Drawing for the job (mm, zero at the part's lowest x, y, z). A direction names the side the tool comes from. Give positions to 0.01 mm unless a question says otherwise; leave off trailing zeros. Order: outer loops, then holes, each group sorted by start corner. A loop starts at its lowest first (then second) coordinate and runs counter-clockwise, first axis right, second up. Notation, with made-up numbers: (43.25, 17.25) - (53.25, 17.25) arc R20 ccw to (53.25, 25.25) - close; hole circle Ø8 at (62.5, 49.25). An arc over 180 degrees is marked (long way). Use a Markdown table: item, result. Add a question column.
(1) Slice it at A-A (y = 12). Write the cut outline in (x, z) (1 decimal).
(2) Which spindle directions (+Z, -Z, +X, -X, +Y, -Y) get a long thin tool onto all of the face, cutting with end or side? Do the marked faces 1, 2 and 3. Say none if no direction does.
(3) Slice it at B-B (x = 4.45). Write the cut outline in (y, z) (1 decimal), then the cut area to 3 significant figures.
(4) Wall check: line 1 (Z direction, x = 0.5, y = 5.75) (1 decimal). Give the ranges that are in metal, low to high.
(5) Slice it at C-C (z = 4.45). Write the cut outline in (x, y) (1 decimal), then the cut area to 3 significant figures.
(6) Flat gauge pins, fed straight in: pin 1 (0.8 mm diameter, centred on y = 11, z = 4, fed in from +X) (1 decimal); pin 2 (0.8 mm diameter, centred on x = 1, y = 7, fed in from -Z); pin 3 (0.8 mm diameter, centred on x = 1, y = 7, fed in from +Z) (1 decimal). Where does each tip first touch, or does it go through?
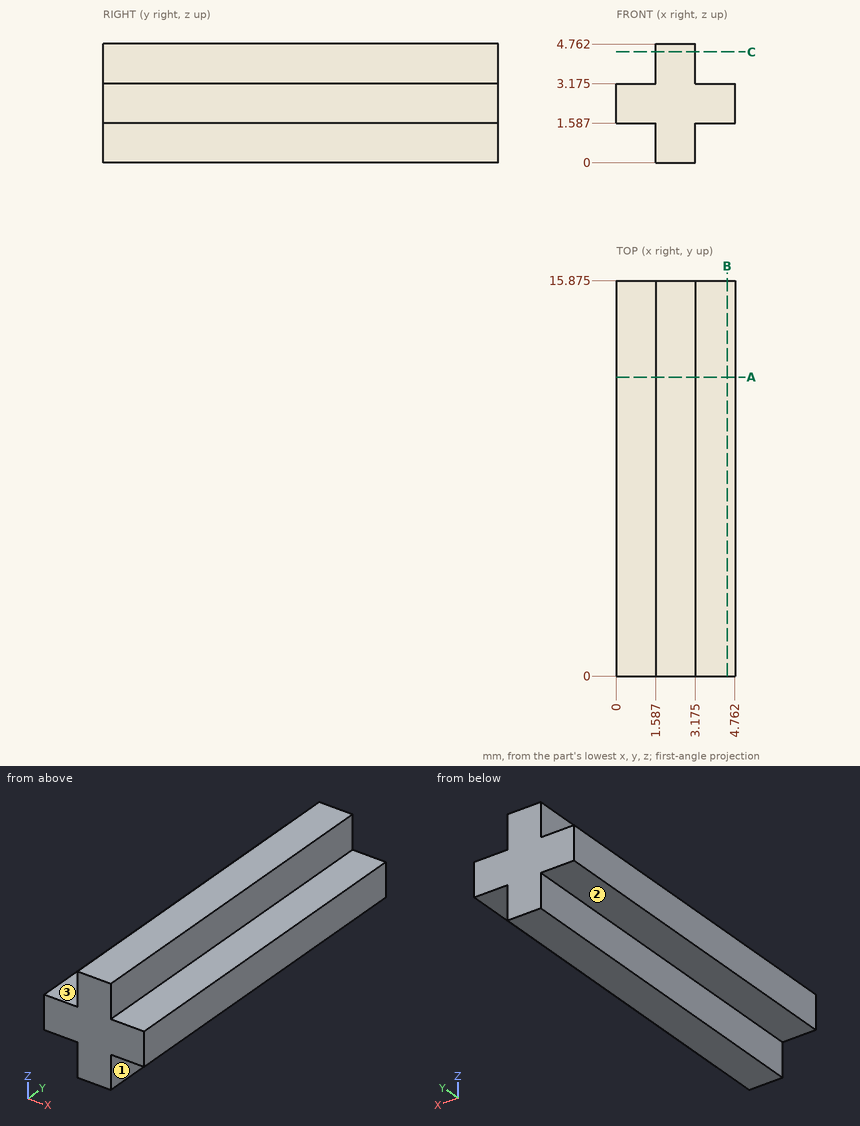
Solution:
| question | item | result |
|---|---|---|
| 1 | outline | (0, 1.6) - (1.6, 1.6) - (1.6, 0) - (3.2, 0) - (3.2, 1.6) - (4.8, 1.6) - (4.8, 3.2) - (3.2, 3.2) - (3.2, 4.8) - (1.6, 4.8) - (1.6, 3.2) - (0, 3.2) - close |
| 2 | face 1 | -Z, +X, +Y, -Y |
| 2 | face 2 | -Z, -X, +Y, -Y |
| 2 | face 3 | +Z, -X, +Y, -Y |
| 3 | outline | (0, 1.6) - (15.9, 1.6) - (15.9, 3.2) - (0, 3.2) - close |
| 3 | area | 25.2 mm2 |
| 4 | line 1 | 1.6 to 3.2 |
| 5 | outline | (1.6, 0) - (3.2, 0) - (3.2, 15.9) - (1.6, 15.9) - close |
| 5 | area | 25.2 mm2 |
| 6 | pin 1 | x = 3.2 |
| 6 | pin 2 | z = 1.59 |
| 6 | pin 3 | z = 3.2 |
